Can you work these out from the model? Positions are in its coordinate system, mm. Face numbers are marked on the shaded views. A direction names the side the tool comes from. Round coordinates to 2 decimals unless told otherwise and drop trailing zeros. Loops run counter-clockwise (first coordinate to the right, second up) from the corner with the lowest first, then second, coordinate; pieces in that order, holes last.
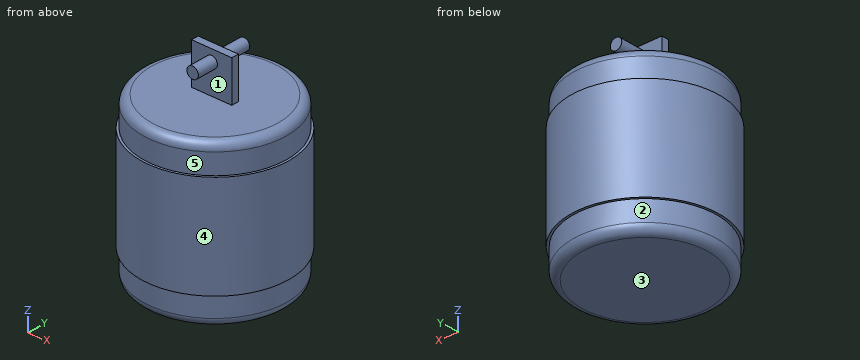
from build123d import *

# Parameters (mm, degrees)
SKETCH1_R                = 18
BOSS_EXTRUDE3_DEPTH      = 25
SKETCH2_R                = 17.45
BOSS_EXTRUDE4_DEPTH      = 7
BOSS_EXTRUDE5_START      = -25
SKETCH2_2_R              = 17.45
BOSS_EXTRUDE5_DEPTH      = 7
FILLET1_R                = 2
FILLET2_R                = 2
SKETCH7_W                = 9.836471502
SKETCH7_H                = 1.801063134
BOSS_EXTRUDE7_DEPTH      = 10
SKETCH8_R                = 1.4
BOSS_EXTRUDE9_DEPTH      = 7
BOSS_EXTRUDE9_DEPTH_BACK = 7


with BuildPart() as part:
    # Sketch1 → Boss-Extrude3 (new body)
    with BuildSketch(Plane.XY):
        Circle(SKETCH1_R)
    extrude(amount=BOSS_EXTRUDE3_DEPTH)

    # Sketch2 → Boss-Extrude4 (add)
    with BuildSketch(Plane.XY.offset(25)):
        Circle(SKETCH2_R)
    extrude(amount=BOSS_EXTRUDE4_DEPTH)

    # Sketch2_2 → Boss-Extrude5 (add)
    with BuildSketch(Plane.XY.offset(25).offset(BOSS_EXTRUDE5_START)):
        Circle(SKETCH2_2_R)
    extrude(amount=-BOSS_EXTRUDE5_DEPTH)

    # Fillet1
    fillet1_edges = [part.edges().sort_by_distance(p)[0] for p in [
        (-17.45, 0, 32),
    ]]
    fillet(fillet1_edges, radius=FILLET1_R)

    # Fillet2
    fillet2_edges = [part.edges().sort_by_distance(p)[0] for p in [
        (-17.45, 0, -7),
    ]]
    fillet(fillet2_edges, radius=FILLET2_R)

    # Sketch7 → Boss-Extrude7 (add)
    with BuildSketch(Plane.XY.offset(32)):
        Rectangle(SKETCH7_W, SKETCH7_H)
    extrude(amount=BOSS_EXTRUDE7_DEPTH)

    # Sketch8 → Boss-Extrude9 (add, two sides)
    with BuildSketch(Plane(origin=(0, 0.900531567, 0), x_dir=(1, 0, 0), z_dir=(0, 1, 0))) as boss_extrude9_sk:
        with Locations((0, -39.2)):
            Circle(SKETCH8_R)
    extrude(amount=BOSS_EXTRUDE9_DEPTH)
    extrude(boss_extrude9_sk.sketch, amount=-BOSS_EXTRUDE9_DEPTH_BACK)


solid = part.part
(1) If I drill on line 1 (Z direction, x = -12.5, y = -5); line 2 (Y direction, x = -2.5, z = 35); line 3 (X direction, y = -0.5, z = 13), over which ranges is the centre line in solid material (lowest first)?
Worked answers:
line 1: z = -7 to 32
line 2: y = -0.9 to 0.9
line 3: x = -17.99 to 17.99
(2) If we section it at A-A, the plane x = 0: List the corners of the cut face in (y, z) for me.
Worked answers:
outline: (-18, 0) - (-17.45, 0) - (-17.45, -5) arc R2 ccw to (-15.45, -7) - (15.45, -7) arc R2 ccw to (17.45, -5) - (17.45, 0) - (18, 0) - (18, 25) - (17.45, 25) - (17.45, 30) arc R2 ccw to (15.45, 32) - (0.9, 32) - (0.9, 37.8) - (7.9, 37.8) - (7.9, 40.6) - (0.9, 40.6) - (0.9, 42) - (-0.9, 42) - (-0.9, 40.6) - (-6.1, 40.6) - (-6.1, 37.8) - (-0.9, 37.8) - (-0.9, 32) - (-15.45, 32) arc R2 ccw to (-17.45, 30) - (-17.45, 25) - (-18, 25) - close
(3) If we section it at C-C, the plane z = 6: List the corners of the cut face in (x, y) for me.
Worked answers:
outline: circle Ø36 at (0, 0)
(4) If we mould it in two halves opening along Z, with no side actions, what happens to the marked faces 1, 2 and 3? For each: released by +Z, released by -Z, zero draft, split by the parting line, or undercut.
Worked answers:
face 1: undercut
face 2: zero draft
face 3: released by -Z
(5) Will these pins go through, and if not, where does the flat tip stop? P1, Ø1.5, axis at x = -4, z = 22.5, coming from the -Y side; P2, Ø6, axis at x = 7, z = 25.5, coming from the -Y side; P3, Ø5, axis at x = 2, z = 36.5, coming from the -Y side.
Worked answers:
P1: stops at y = -17.7
P2: stops at y = -17.54
P3: stops at y = -6.1
(6) If we section it at D-D, the plane z = 29: List the corners of the cut face in (x, y) for me.
Worked answers:
outline: circle Ø34.9 at (0, 0)
(7) If we section it at B-B, the plane y = 0: List the corners of the cut face in (x, z) for me, then the cut area to 3 significant figures.
Worked answers:
outline: (-18, 0) - (-17.45, 0) - (-17.45, -5) arc R2 ccw to (-15.45, -7) - (15.45, -7) arc R2 ccw to (17.45, -5) - (17.45, 0) - (18, 0) - (18, 25) - (17.45, 25) - (17.45, 30) arc R2 ccw to (15.45, 32) - (4.92, 32) - (4.92, 42) - (-4.92, 42) - (-4.92, 32) - (-15.45, 32) arc R2 ccw to (-17.45, 30) - (-17.45, 25) - (-18, 25) - close
area: 1,480 mm2
(8) For the marked faces 4 and 5, which set-ups out of +Z, -Z, +X, -X, +Y, -Y let a thin tool reach every point of the face, with its end or its side?
Worked answers:
face 4: +Z, -Z
face 5: +Z
